from build123d import *

# Parameters (mm, degrees)
SKETCH1_W           = 125
SKETCH1_H           = 84
BOSS_EXTRUDE1_DEPTH = 2.85
SKETCH2_R           = 1.5
CUT_EXTRUDE1_DEPTH  = 76.354976611
SKETCH3_R           = 2.4
CUT_EXTRUDE2_DEPTH  = 76.354976611
SKETCH4_R           = 1.7
SKETCH4_W           = 2.85
SKETCH4_H           = 10
CUT_EXTRUDE3_DEPTH  = 76.354976611
SKETCH5_R           = 1.7
SKETCH5_W           = 10
SKETCH5_H           = 2.85
CUT_EXTRUDE4_DEPTH  = 76.354976611
SKETCH6_W           = 50
SKETCH6_H           = 56
CUT_EXTRUDE5_DEPTH  = 76.354976611
FILLET1_R           = 6


with BuildPart() as part:
    # Sketch1 → Boss-Extrude1 (new body)
    with BuildSketch(Plane(origin=(0, 0, 0), x_dir=(1, 0, 0), z_dir=(0, 1, 0))):
        Rectangle(SKETCH1_W, SKETCH1_H)
    extrude(amount=BOSS_EXTRUDE1_DEPTH)

    # Sketch2 → Cut-Extrude1 (cut, through all)
    with BuildSketch(Plane.XZ):
        with Locations(Location((44.5, 0, 0), (0, 0, 270))):
            Circle(SKETCH2_R)
    extrude(amount=-CUT_EXTRUDE1_DEPTH, mode=Mode.SUBTRACT)

    # Sketch3 → Cut-Extrude2 (cut, through all)
    with BuildSketch(Plane(origin=(0, 2.85, 0), x_dir=(1, 0, 0), z_dir=(0, 1, 0))):
        with Locations(Location((-26.6, 0, 0), (0, 0, 270))):
            Circle(SKETCH3_R)
        with Locations(Location((-26.6, 37.5, 0), (0, 0, 270))):
            Circle(SKETCH3_R)
        with Locations(Location((-26.6, -37.5, 0), (0, 0, 270))):
            Circle(SKETCH3_R)
    extrude(amount=-CUT_EXTRUDE2_DEPTH, mode=Mode.SUBTRACT)

    # Sketch4 → Cut-Extrude3 (cut, through all)
    with BuildSketch(Plane(origin=(0, 2.85, 0), x_dir=(1, 0, 0), z_dir=(0, 1, 0))):
        with Locations((-61.075, -19.25)):
            Circle(SKETCH4_R)
        with Locations((-61.075, 19.25)):
            Circle(SKETCH4_R)
        with Locations((-61.075, 0)):
            Rectangle(SKETCH4_W, SKETCH4_H)
    extrude(amount=-CUT_EXTRUDE3_DEPTH, mode=Mode.SUBTRACT)

    # Sketch5 → Cut-Extrude4 (cut, through all)
    with BuildSketch(Plane(origin=(0, 2.85, 0), x_dir=(1, 0, 0), z_dir=(0, 1, 0))):
        with Locations((37.5, 40.575)):
            Circle(SKETCH5_R)
        with Locations((52.5, 40.575)):
            Rectangle(SKETCH5_W, SKETCH5_H)
        with Locations((22.5, 40.575)):
            Rectangle(SKETCH5_W, SKETCH5_H)
    cut_extrude4 = extrude(amount=-CUT_EXTRUDE4_DEPTH, mode=Mode.SUBTRACT)

    # Mirror1: Cut-Extrude4 across plane
    add(cut_extrude4.mirror(Plane.XY), mode=Mode.SUBTRACT)

    # Sketch6 → Cut-Extrude5 (cut, through all)
    with BuildSketch(Plane(origin=(0, 2.85, 0), x_dir=(1, 0, 0), z_dir=(0, 1, 0))):
        with Locations((37.5, 0)):
            Rectangle(SKETCH6_W, SKETCH6_H)
    extrude(amount=-CUT_EXTRUDE5_DEPTH, mode=Mode.SUBTRACT)

    # Fillet1
    fillet1_edges = [part.edges().sort_by_distance(p)[0] for p in [
        (62.5, 1.425, -28),
        (62.5, 1.425, 28),
        (12.5, 1.425, 28),
        (12.5, 1.425, -28),
    ]]
    fillet(fillet1_edges, radius=FILLET1_R)


solid = part.part
Design review of the part built by this model. Coordinates are the model's own, in mm. A direction names the side the tool comes from. Round coordinates to 2 decimals unless told otherwise and drop trailing zeros. Write each loop counter-clockwise with the first axis right and the second up, starting at its lowest first coordinate (ties: lowest second). Pieces come first, ordered by that corner, then holes. Notation, with made-up numbers: (87.5, -23) -> (104.5, -23) arc R28 cw to (104.5, 6) -> close; hole circle Ø9 at (50.5, 6.5). An arc over 180 degrees is marked (long way). One line per question, with ' | ' between items.
(1) Machinability: for faces 5 (the flat face through (22, 1, -39.15)), 6 (the cylindrical face through (14.211, 1.405, 26.196)), 7 (the flat face through (17.5, 1, 41)), which of the approach directions +Z, -Z, +X, -X, +Y, -Y give a long, thin tool a straight path to every point of the face, cutting with its end or side? Answer none if there is none.
Result sheet:
face 5: -Z, +Y, -Y | face 6: +X, +Y, -Y | face 7: +Z, +Y, -Y
(2) Wall thickness on line 1 (Z direction, x = 57, y = 1.3); line 2 (X direction, y = 2.65, z = -37.5); line 3 (X direction, y = 1.05, z = 13): over which ranges is each line inside the solid? List them lowest first. Write a range as [from, to].
Result sheet:
line 1: [-39.15, -28.02], [28.02, 39.15] | line 2: [-62.5, -29], [-24.2, 62.5] | line 3: [-62.5, 12.5]
(3) Take a section at C-C, the plane y = 2.1. State how many separate pieces and enclosed holes the cut face has, and give its area (3 significant figures).
Result sheet:
separate pieces: 1 | enclosed holes: 3 | area: 7,470 mm2
(4) Take a section at D-D, the plane z = 37.5. State the section outline as (x, y) points.
Result sheet:
outline: (-62.5, 0) -> (-29, 0) -> (-29, 2.85) -> (-62.5, 2.85) -> close; (-24.2, 0) -> (62.5, 0) -> (62.5, 2.85) -> (-24.2, 2.85) -> close
(5) Take a section at A-A, the plane z = 0. State the section outline as (x, y) points.
Result sheet:
outline: (-59.65, 0) -> (-29, 0) -> (-29, 2.85) -> (-59.65, 2.85) -> close; (-24.2, 0) -> (12.5, 0) -> (12.5, 2.85) -> (-24.2, 2.85) -> close
(6) Insertion check: P1, Ø4.5, axis at x = -26.6, z = 37.5, coming from the -Y side; P2, Ø0.9, axis at x = 24.5, y = 1, coming from the +Z side. Each pin has a flat end and moves straight along its axis. Give the tip position at first contact, or say it passes through.
Result sheet:
P1: through | P2: z = 39.15
(7) Take a section at B-B, the plane x = -26.6. State the section outline as (y, z) points, and give its area (3 significant figures).
Result sheet:
outline: (0, -42) -> (2.85, -42) -> (2.85, -39.9) -> (0, -39.9) -> close; (0, -35.1) -> (2.85, -35.1) -> (2.85, -2.4) -> (0, -2.4) -> close; (0, 2.4) -> (2.85, 2.4) -> (2.85, 35.1) -> (0, 35.1) -> close; (0, 39.9) -> (2.85, 39.9) -> (2.85, 42) -> (0, 42) -> close | area: 198 mm2
(8) Draft analysis for pull direction Z (two halves, no side actions). For faces 1 (the flat face through (-62.5, 1, 31)), 2 (the flat face through (12.5, 1, 0)), 3 (the flat face through (43, 1, -42)), 4 (the flat face through (37, 1, -28)), state which applies: released by +Z, released by -Z, zero draft, split by the parting line, or undercut.
Result sheet:
face 1: zero draft | face 2: undercut | face 3: released by -Z | face 4: undercut
